The drawing under review shows one solid part. Ordinate dimensions are in mm from its lowest x, y, z. A direction names the side the tool comes from. Coordinates: 2 decimals unless noted, no trailing zeros. Write each loop counter-clockwise with the first axis right and the second up, starting at its lowest first coordinate (ties: lowest second). Pieces come first, ordered by that corner, then holes.
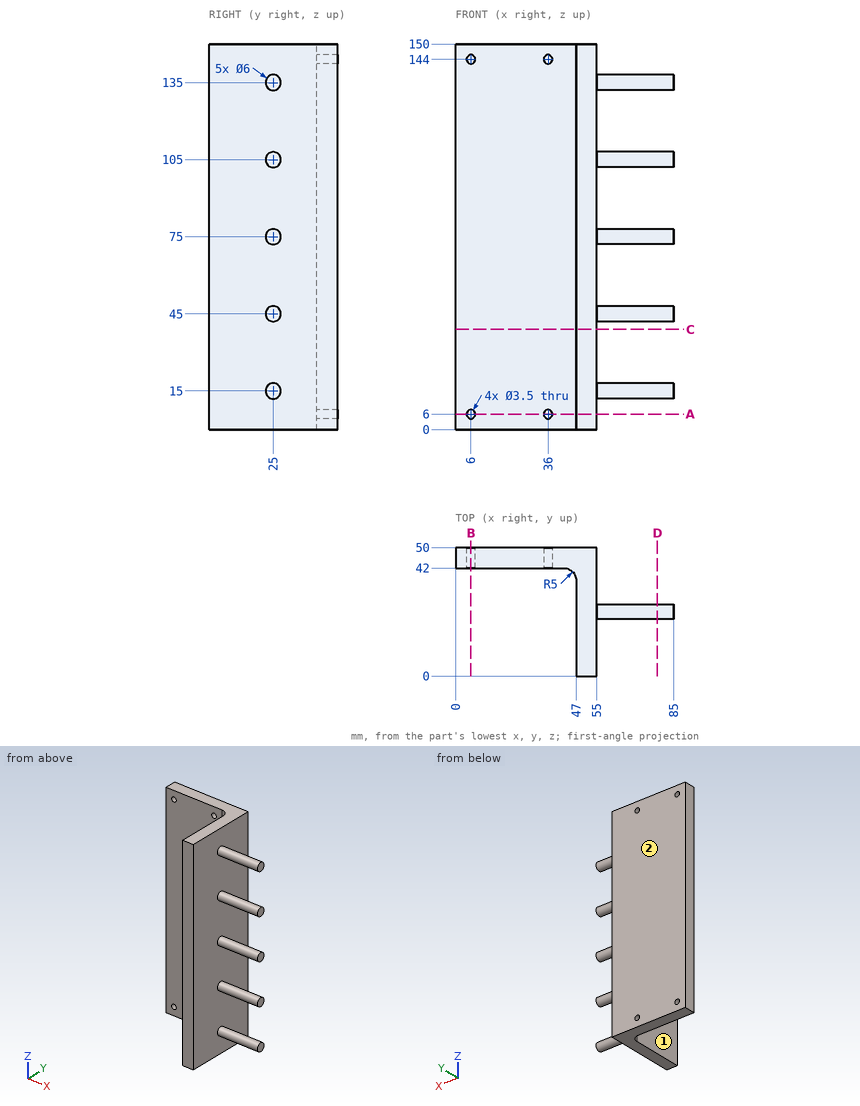
1) Tool access review of the marked faces 1 and 2: name each direction out of +Z, -Z, +X, -X, +Y, -Y from which nothing blocks a thin tool from reaching the whole face with its end or side.
2) Clearance check with flat-ended pins moving along their axes: P1, Ø2, axis at y = 30, z = 98, coming from the -X side; P2, Ø4.5, axis at x = 36, z = 6, coming from the -Y side; P3, Ø25, axis at y = 28, z = 92, coming from the +X side. State where each tip first meets the part, or that it passes through.
3) Consider section B-B (x = 6). Give the boundary of the cut face in (y, z), then the cut area to 3 significant figures.
4) Consider section D-D (x = 78.5). Give the boundary of the cut face in (y, z).
5) For L1, parallel to Z at x = 36, y = 45; L2, parallel to X at y = 48, z = 144; L3, parallel to X at y = 46.5, z = 142.5, list the stretches that pass through material, from the lowest coordinate up.
6) Consider section A-A (z = 6). Give the boundary of the cut face in (x, y).
7) Consider section C-C (z = 39). Give the boundary of the cut face in (x, y).
Results:
1. face 1: +Z, -Z, -X, -Y
1. face 2: +Z, -Z, +X, -X, +Y
2. P1: stops at x = 47
2. P2: stops at y = 42
2. P3: stops at x = 85
3. outline: (42, 0) - (50, 0) - (50, 4.25) - (42, 4.25) - close; (42, 7.75) - (50, 7.75) - (50, 142.25) - (42, 142.25) - close; (42, 145.75) - (50, 145.75) - (50, 150) - (42, 150) - close
3. area: 1,140 mm2
4. outline: circle Ø6 at (25, 15); circle Ø6 at (25, 45); circle Ø6 at (25, 75); circle Ø6 at (25, 105); circle Ø6 at (25, 135)
5. L1: z = 0 to 4.25, 7.75 to 142.25, 145.75 to 150
5. L2: x = 0 to 4.25, 7.75 to 34.25, 37.75 to 55
5. L3: x = 0 to 5.1, 6.9 to 35.1, 36.9 to 55
6. outline: (0, 42) - (4.25, 42) - (4.25, 50) - (0, 50) - close; (7.75, 42) - (34.25, 42) - (34.25, 50) - (7.75, 50) - close; (37.75, 42) - (42, 42) arc R5 cw to (47, 37) - (47, 0) - (55, 0) - (55, 50) - (37.75, 50) - close
7. outline: (0, 42) - (42, 42) arc R5 cw to (47, 37) - (47, 0) - (55, 0) - (55, 50) - (0, 50) - close
